```python
from build123d import *

# Parameters (mm, degrees)
F0_R     = 6.870187
F0_R_2   = 1.25
F1_DEPTH = 1.8


with BuildPart() as f1:
    # F0 (on Front) → F1 (new body)
    with BuildSketch(Plane.XZ):
        Circle(F0_R)
        with BuildLine():
            ThreePointArc((4.565355, 3.022111), (5.242659, 1.578022), (5.475, 0))
            ThreePointArc((5.475, 0), (4.037518, -3.697847), (0.479905, -5.453927))
            ThreePointArc((0.479905, -5.453927), (-0.080045, -5.474415), (-0.639157, -5.437564))
            ThreePointArc((-0.639157, -5.437564), (-4.916584, -2.408906), (-4.688537, 2.827233))
            ThreePointArc((-4.688537, 2.827233), (-4.515673, 3.095855), (-4.327438, 3.353939))
            ThreePointArc((-4.327438, 3.353939), (-0.165763, 5.47249), (4.116508, 3.609708))
            ThreePointArc((4.116508, 3.609708), (4.350862, 3.323495), (4.565355, 3.022111))
        make_face(mode=Mode.SUBTRACT)
        with BuildLine():
            ThreePointArc((2.75, 0), (2.654061, 0.720041), (2.372939, 1.389842))
            ThreePointArc((2.372939, 1.389842), (2.161642, 1.699942), (1.910097, 1.978391))
            ThreePointArc((1.910097, 1.978391), (-0.062718, 2.749285), (-1.998327, 1.88923))
            ThreePointArc((-1.998327, 1.88923), (-2.287733, 1.526034), (-2.511897, 1.119318))
            ThreePointArc((-2.511897, 1.119318), (-2.377631, -1.3818), (-0.270954, -2.736619))
            ThreePointArc((-0.270954, -2.736619), (0, -2.75), (0.270954, -2.736619))
            ThreePointArc((0.270954, -2.736619), (2.03809, -1.846263), (2.75, 0))
        make_face()
        Circle(F0_R_2, mode=Mode.SUBTRACT)
        with BuildLine():
            Line((2.372939, 1.389842), (4.565355, 3.022111))
            ThreePointArc((4.565355, 3.022111), (4.350862, 3.323495), (4.116508, 3.609708))
            Line((4.116508, 3.609708), (1.910097, 1.978391))
            ThreePointArc((1.910097, 1.978391), (2.161642, 1.699942), (2.372939, 1.389842))
        make_face()
        with BuildLine():
            ThreePointArc((-0.639157, -5.437564), (-0.080045, -5.474415), (0.479905, -5.453927))
            Line((0.479905, -5.453927), (0.270954, -2.736619))
            ThreePointArc((0.270954, -2.736619), (0, -2.75), (-0.270954, -2.736619))
            Line((-0.270954, -2.736619), (-0.639157, -5.437564))
        make_face()
        with BuildLine():
            Line((-1.998327, 1.88923), (-4.327438, 3.353939))
            ThreePointArc((-4.327438, 3.353939), (-4.515673, 3.095855), (-4.688537, 2.827233))
            Line((-4.688537, 2.827233), (-2.511897, 1.119318))
            ThreePointArc((-2.511897, 1.119318), (-2.287733, 1.526034), (-1.998327, 1.88923))
        make_face()
    extrude(amount=-F1_DEPTH)


solid = f1.part
```
Check sheet for the modelled part. Datum: model origin and axes. Units: mm. A direction names the side the tool comes from. Coordinates: 2 decimals unless noted, no trailing zeros. Write each loop counter-clockwise with the first axis right and the second up, starting at its lowest first coordinate (ties: lowest second). Pieces come first, ordered by that corner, then holes. Notation, with made-up numbers: M 44.5,48 L 79.5,48 A21 cw 79.5,63 Z; hole C -2,-37 d8. An arc over 180 degrees is marked long. Write item = value, one per line. Start each with the question number.
1. Thickness scan on probe 1 along Z at (x, y) = (0, 1.1) (3 decimals); probe 2 along Z at (x, y) = (3.25, 0.8); probe 3 along X at (y, z) = (0.9, -4.25). Record the ranges inside material, lowest first.
2. Mould release check, pull along X, two halves, no side actions. Record for faces 1 (the flat face through (-3.62, 0.89, 1.99)), 2 (the flat face through (-0.1, 1.8, -1.4)), 3 (the cylindrical face through (6.553, 0.887, 2.064)), 4 (the flat face through (-3.147, 0.887, 2.611)): pulls with the +X half, pulls with the -X half, needs draft (parallel to the pull), parting line crosses it, or undercut.
3. Sectioned sample at A-A (x = 0). Record the cut outline in (y, z) (3 decimals).
4. Sectioned sample at C-C (z = 5.25). Record the cut outline in (x, y).
5. Tool access check on faces 5 (the cylindrical face through (-4.88, 0.89, -2.48)), 6 (the flat face through (-0.1, 0, -1.4)). Record the directions out of +Z, -Z, +X, -X, +Y, -Y that give a thin tool (end or side, any length) a straight path to the whole face; none if there is none.
6. Sectioned sample at B-B (y = 1.5). State how many separate pieces and enclosed holes the cut face has, then the cut area to 3 significant figures.
7. Sectioned sample at D-D (z = -4). Record the cut outline in (x, y), then the cut area to 3 significant figures.
8. Go/stop test with flat-tipped pins: pin 1 (1 mm diameter, centred on x = 4, y = 1, fed in from +Z); pin 2 (1 mm diameter, centred on y = 1.5, z = -5, fed in from +X); pin 3 (1 mm diameter, centred on y = 0.5, z = 1.5, fed in from -X). Record where each tip stops, or that it passes through.
The answers:
q1.probe_1 = -6.87 to -1.25, 1.25 to 2.75, 5.475 to 6.87
q1.probe_2 = -6.05 to -4.41, 2.04 to 2.97, 4.41 to 6.05
q1.probe_3 = -5.4 to -3.45, -0.48 to 0.39, 3.45 to 5.4
q2.face_1 = undercut
q2.face_2 = needs draft
q2.face_3 = parting line crosses it
q2.face_4 = undercut
q3.outline = M 0,-6.87 L 1.8,-6.87 L 1.8,-1.25 L 0,-1.25 Z; M 0,1.25 L 1.8,1.25 L 1.8,2.75 L 0,2.75 Z; M 0,5.475 L 1.8,5.475 L 1.8,6.87 L 0,6.87 Z
q4.outline = M -4.43,0 L -1.55,0 L -1.55,1.8 L -4.43,1.8 Z; M 1.55,0 L 4.43,0 L 4.43,1.8 L 1.55,1.8 Z
q5.face_5 = +Y, -Y
q5.face_6 = +Z, -Z, +X, -X, -Y
q6.separate_pieces = 1
q6.enclosed_holes = 4
q6.area = 79.4 mm²
q7.outline = M -5.59,0 L -3.74,0 L -3.74,1.8 L -5.59,1.8 Z; M -0.44,0 L 0.37,0 L 0.37,1.8 L -0.44,1.8 Z; M 3.74,0 L 5.59,0 L 5.59,1.8 L 3.74,1.8 Z
q7.area = 8.11 mm²
q8.pin_1 = 5.91
q8.pin_2 = 5.19
q8.pin_3 = -6.8
